Here's the drawing with two shaded views (mm, measured from the low corner). I have some questions. A direction names the side the tool comes from. Round coordinates to 2 decimals unless told otherwise and drop trailing zeros. Loops run counter-clockwise (first coordinate to the right, second up) from the corner with the lowest first, then second, coordinate; pieces in that order, holes last.
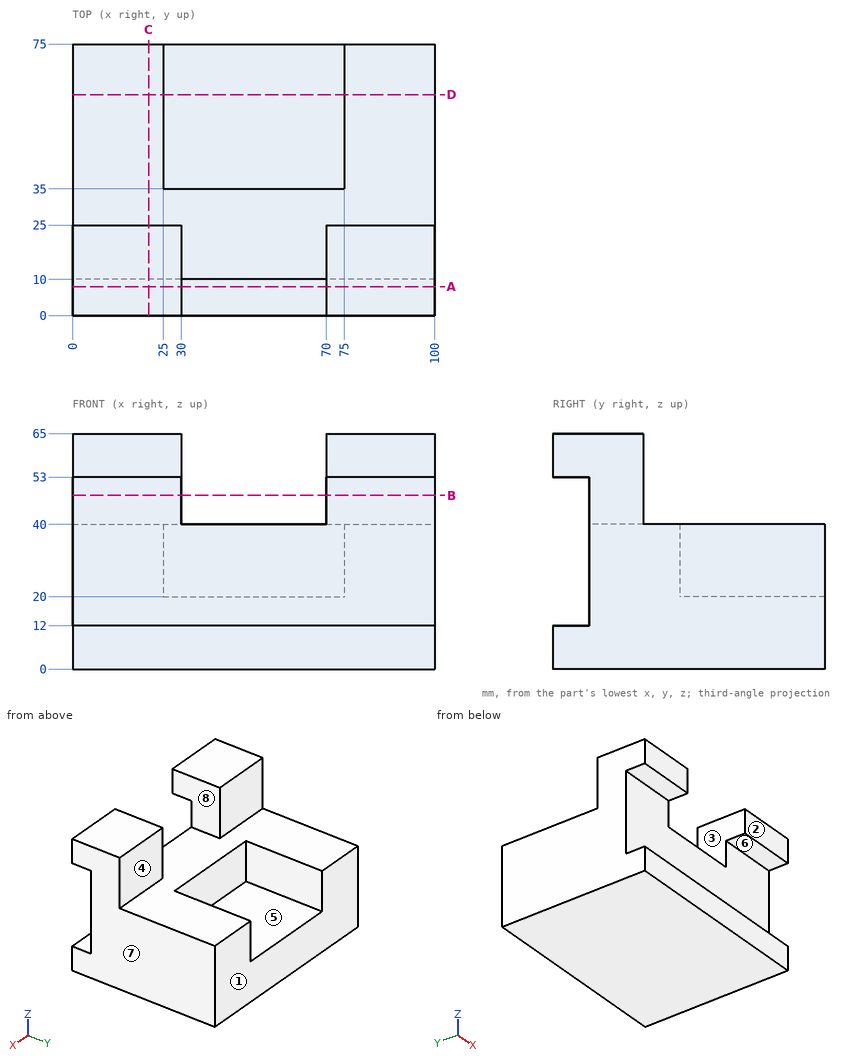
Item 1: Will these pins go through, and if not, where does the flat tip stop? pin 1 (12 mm diameter, centred on x = 48, y = 16, fed in from +Z); pin 2 (6 mm diameter, centred on x = 56, z = 29.5, fed in from +Y); pin 3 (12.5 mm diameter, centred on x = 80, z = 52, fed in from +Y).
Results list:
pin 1: stops at z = 40
pin 2: stops at y = 35
pin 3: stops at y = 25
Item 2: For the marked faces 4, 5, 6, 7 and 8, which set-ups out of +Z, -Z, +X, -X, +Y, -Y let a thin tool reach every point of the face, with its end or its side?
Results list:
face 4: +Z, +X, -X, +Y
face 5: +Z, +Y
face 6: +X, -X, -Y
face 7: +Z, -Z, +X, +Y, -Y
face 8: +Z, +Y, -Y
Item 3: If we section it at C-C, the plane x = 21: Please give me the cut outline in (y, z).
Results list:
outline: (0, 0) - (75, 0) - (75, 40) - (25, 40) - (25, 65) - (0, 65) - (0, 53) - (10, 53) - (10, 12) - (0, 12) - close
Item 4: If we section it at D-D, the plane y = 61: Please give me the cut outline in (x, z), then the cut area to 3 significant figures.
Results list:
outline: (0, 0) - (100, 0) - (100, 40) - (75, 40) - (75, 20) - (25, 20) - (25, 40) - (0, 40) - close
area: 3,000 mm2
Item 5: If we section it at B-B, the plane z = 48: Please give me the cut outline in (x, y).
Results list:
outline: (0, 10) - (30, 10) - (30, 25) - (0, 25) - close; (70, 10) - (100, 10) - (100, 25) - (70, 25) - close
Item 6: If we section it at A-A, the plane y = 8: Please give me the cut outline in (x, z).
Results list:
outline: (0, 0) - (100, 0) - (100, 12) - (0, 12) - close; (0, 53) - (30, 53) - (30, 65) - (0, 65) - close; (70, 53) - (100, 53) - (100, 65) - (70, 65) - close
Item 7: We'd pull the mould along Y, two halves only. Please class the marked faces 1, 2 and 3: released by +Y, released by -Y, zero draft, split by the parting line, or undercut.
Results list:
face 1: released by +Y
face 2: released by -Y
face 3: zero draft
Item 8: If I drill on line 1 along X through (y, z) = (51, 34); line 2 along Z through (x, y) = (37, 42); line 3 along Y through (x, z) = (72, 45.5), over which ranges is the centre line in solid material (lowest first)?
Results list:
line 1: x = 0 to 25, 75 to 100
line 2: z = 0 to 20
line 3: y = 10 to 25
